Build history of the part. All positions in model axes, mm. Give positions to 0.01 mm unless a question says otherwise; leave off trailing zeros. Write each loop counter-clockwise with the first axis right and the second up, starting at its lowest first coordinate (ties: lowest second). Pieces come first, ordered by that corner, then holes.
from build123d import *

# Parameters (mm, degrees)
IZIM1_R                     = 1.5
Y_KSEKLIK_EKSTR_ZYON1_DEPTH = 1.6


with BuildPart() as part:
    # Çizim1 → Yükseklik-Ekstrüzyon1 (new body)
    with BuildSketch(Plane.XY):
        with BuildLine():
            Line((51.878679656, -0.878679656), (62.901413512, -11.901413512))
            ThreePointArc((62.901413512, -11.901413512), (63.179114484, -12.782168471), (62.616924992, -13.51482808))
            Line((62.616924992, -13.51482808), (61.615557944, -13.981773203))
            ThreePointArc((61.615557944, -13.981773203), (60.959512838, -14.047839782), (60.404952381, -13.691156907))
            ThreePointArc((60.404952381, -13.691156907), (53.799180994, -16.856750014), (61.123557768, -16.753308252))
            ThreePointArc((61.123557768, -16.753308252), (61.318334892, -16.334489822), (61.680554911, -16.047882666))
            Line((61.680554911, -16.047882666), (63.577381738, -15.16337779))
            ThreePointArc((63.577381738, -15.16337779), (64.537299608, -15.226294131), (65, -16.069685577))
            Line((65, -16.069685577), (65, -29))
            ThreePointArc((65, -29), (64.414213562, -30.414213562), (63, -31))
            Line((63, -31), (57.505773979, -31))
            ThreePointArc((57.505773979, -31), (55.962548796, -30.572636009), (54.859002861, -29.412304022))
            ThreePointArc((54.859002861, -29.412304022), (32.5, -16), (10.140997139, -29.412304022))
            ThreePointArc((10.140997139, -29.412304022), (9.037451204, -30.572636009), (7.494226021, -31))
            Line((7.494226021, -31), (2, -31))
            ThreePointArc((2, -31), (0.585786438, -30.414213562), (0, -29))
            Line((0, -29), (0, -16.069685577))
            ThreePointArc((0, -16.069685577), (0.462700392, -15.226294131), (1.422618262, -15.16337779))
            Line((1.422618262, -15.16337779), (3.319445089, -16.047882666))
            ThreePointArc((3.319445089, -16.047882666), (3.681665108, -16.334489822), (3.876442232, -16.753308252))
            ThreePointArc((3.876442232, -16.753308252), (11.200819006, -16.856750014), (4.595047619, -13.691156907))
            ThreePointArc((4.595047619, -13.691156907), (4.040487162, -14.047839782), (3.384442056, -13.981773203))
            Line((3.384442056, -13.981773203), (2.383075008, -13.51482808))
            ThreePointArc((2.383075008, -13.51482808), (1.820885516, -12.782168471), (2.098586488, -11.901413512))
            Line((2.098586488, -11.901413512), (13.121320344, -0.878679656))
            ThreePointArc((13.121320344, -0.878679656), (14.09459039, -0.228361402), (15.242640687, 0))
            Line((15.242640687, 0), (30.55, 0))
            ThreePointArc((30.55, 0), (31.257106781, -0.292893219), (31.55, -1))
            Line((31.55, -1), (31.55, -1.418718434))
            ThreePointArc((31.55, -1.418718434), (31.389799475, -1.961615148), (30.960526316, -2.330567185))
            ThreePointArc((30.960526316, -2.330567185), (32.5, -9.5), (34.039473684, -2.330567185))
            ThreePointArc((34.039473684, -2.330567185), (33.610200525, -1.961615148), (33.45, -1.418718434))
            Line((33.45, -1.418718434), (33.45, -1))
            ThreePointArc((33.45, -1), (33.742893219, -0.292893219), (34.45, 0))
            Line((34.45, 0), (49.757359313, 0))
            ThreePointArc((49.757359313, 0), (50.90540961, -0.228361402), (51.878679656, -0.878679656))
        make_face()
        with Locations((21.25, -11)):
            Circle(IZIM1_R, mode=Mode.SUBTRACT)
        with Locations((43.75, -11)):
            Circle(IZIM1_R, mode=Mode.SUBTRACT)
    extrude(amount=Y_KSEKLIK_EKSTR_ZYON1_DEPTH)


solid = part.part
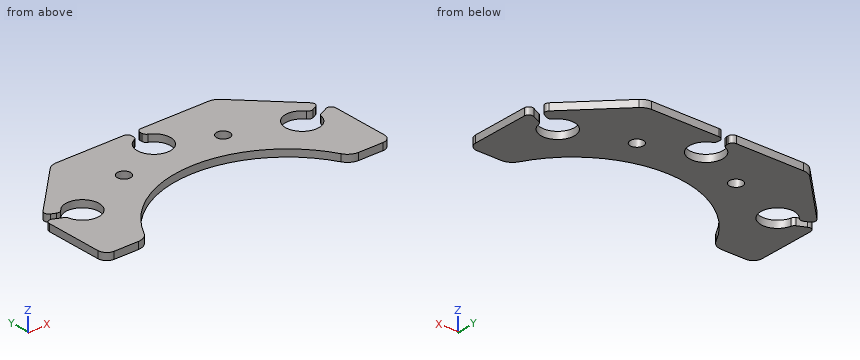
1. Drop flat-ended pins along their axis: pin 1 (0.5 mm diameter, centred on y = -1, z = 1, fed in from -X); pin 2 (2.5 mm diameter, centred on x = 21.25, y = -11, fed in from +Z). Give the stop position or say it passes through.
2. Drill centre lines: line 1 along X through (y, z) = (-13.5, 1.55); line 2 along X through (y, z) = (-7.5, 1.15); line 3 along X through (y, z) = (-12, 1.05). Where is each one in solid material? Low to high.
3. Saw through at D-D on x = 32.5. Give the cut face in (y, z).
4. Saw through at C-C on z = 1.1. Count the separate pieces of the cut face and the enclosed holes in it, plus the area to 3 significant figures.
5. Saw through at B-B on x = 21.25. Give the cut face in (y, z).
6. Saw through at A-A on y = -5.75. Give the cut face in (x, z), plus the area to 3 significant figures.
Outcome:
1. pin 1: stops at x = 12.75
1. pin 2: passes through
2. line 1: x = 2.35 to 4.75, 10.35 to 54.65, 60.25 to 62.65
2. line 2: x = 6.5 to 29.18, 35.82 to 58.5
2. line 3: x = 2.01 to 20.13, 22.37 to 42.63, 44.87 to 62.99
3. outline: (-16, 0) - (-9.5, 0) - (-9.5, 1.6) - (-16, 1.6) - close
4. separate pieces: 1
4. enclosed holes: 2
4. area: 1,150 mm2
5. outline: (-18.63, 0) - (-12.5, 0) - (-12.5, 1.6) - (-18.63, 1.6) - close; (-9.5, 0) - (0, 0) - (0, 1.6) - (-9.5, 1.6) - close
6. outline: (8.25, 0) - (28.75, 0) - (28.75, 1.6) - (8.25, 1.6) - close; (36.25, 0) - (56.75, 0) - (56.75, 1.6) - (36.25, 1.6) - close
6. area: 65.6 mm2
